```python
from build123d import *

# Parameters (mm, degrees)
BASE_SKETCH_W           = 304.8
BASE_SKETCH_H           = 191.39
BOSS_EXTRUDE1_DEPTH     = 11.81
JOINT_X_W               = 25.4
JOINT_X_H               = 11.81
BOSS_EXTRUDE2_DEPTH     = 11.81
JOINT_Y_W               = 11.81
JOINT_Y_H               = 25.4
CUT_EXTRUDE1_DEPTH      = 384.912686042
LPATTERN1_COUNT         = 4
LPATTERN1_PITCH         = 93.133333333
LPATTERN2_COUNT         = 4
LPATTERN2_PITCH         = 59.266666667
MIRROR1_COPY_1_SKETCH_W = 11.81
MIRROR1_COPY_1_SKETCH_H = 25.4
MIRROR1_COPY_1_DEPTH    = 384.912686042
MIRROR1_COPY_2_SKETCH_W = 11.81
MIRROR1_COPY_2_SKETCH_H = 25.4
MIRROR1_COPY_2_DEPTH    = 384.912686042
MIRROR1_COPY_3_SKETCH_W = 11.81
MIRROR1_COPY_3_SKETCH_H = 25.4
MIRROR1_COPY_3_DEPTH    = 384.912686042


with BuildPart() as part:
    # Base_Sketch → Boss-Extrude1 (new body)
    with BuildSketch(Plane.XY):
        with Locations((-199.719002607, -45.012810132)):
            Rectangle(BASE_SKETCH_W, BASE_SKETCH_H)
    extrude(amount=BOSS_EXTRUDE1_DEPTH)

    # Joint_X → Boss-Extrude2 (add)
    with BuildSketch(Plane.XY.offset(11.81)):
        with Locations((-339.419002607, -146.612810132)):
            Rectangle(JOINT_X_W, JOINT_X_H)
    boss_extrude2 = extrude(amount=-BOSS_EXTRUDE2_DEPTH)

    # Joint_Y → Cut-Extrude1 (cut, through all)
    with BuildSketch(Plane.XY.offset(11.81)):
        with Locations((-346.214002607, -139.817810132)):
            Rectangle(JOINT_Y_W, JOINT_Y_H)
    cut_extrude1 = extrude(amount=-CUT_EXTRUDE1_DEPTH, mode=Mode.SUBTRACT)

    # LPattern1: Boss-Extrude2 ×4
    with Locations(*[(i * LPATTERN1_PITCH, 0, 0) for i in range(1, LPATTERN1_COUNT)]):
        add(boss_extrude2)

    # LPattern2: Cut-Extrude1 ×4
    with Locations(*[(0, i * LPATTERN2_PITCH, 0) for i in range(1, LPATTERN2_COUNT)]):
        add(cut_extrude1, mode=Mode.SUBTRACT)

    # Mirror1: Cut-Extrude1 across plane
    add(cut_extrude1.mirror(Plane.ZY.offset(199.719002607)), mode=Mode.SUBTRACT)

    # Mirror1 copy 1 sketch → Mirror1 copy 1 (cut, through all)
    with BuildSketch(Plane(origin=(-399.438005213, 59.266666667, 11.81), x_dir=(-1, 0, 0), z_dir=(0, 0, 1))):
        with Locations((-346.214002607, 139.817810132)):
            Rectangle(MIRROR1_COPY_1_SKETCH_W, MIRROR1_COPY_1_SKETCH_H)
    extrude(amount=-MIRROR1_COPY_1_DEPTH, mode=Mode.SUBTRACT)

    # Mirror1 copy 2 sketch → Mirror1 copy 2 (cut, through all)
    with BuildSketch(Plane(origin=(-399.438005213, 118.533333333, 11.81), x_dir=(-1, 0, 0), z_dir=(0, 0, 1))):
        with Locations((-346.214002607, 139.817810132)):
            Rectangle(MIRROR1_COPY_2_SKETCH_W, MIRROR1_COPY_2_SKETCH_H)
    extrude(amount=-MIRROR1_COPY_2_DEPTH, mode=Mode.SUBTRACT)

    # Mirror1 copy 3 sketch → Mirror1 copy 3 (cut, through all)
    with BuildSketch(Plane(origin=(-399.438005213, 177.8, 11.81), x_dir=(-1, 0, 0), z_dir=(0, 0, 1))):
        with Locations((-346.214002607, 139.817810132)):
            Rectangle(MIRROR1_COPY_3_SKETCH_W, MIRROR1_COPY_3_SKETCH_H)
    extrude(amount=-MIRROR1_COPY_3_DEPTH, mode=Mode.SUBTRACT)


solid = part.part
```
Geometry: final body of the model. Coordinates: model frame, mm. A direction names the side the tool comes from. Round coordinates to 2 decimals unless told otherwise and drop trailing zeros. Order: outer loops, then holes, each group sorted by start corner. A loop starts at its lowest first (then second) coordinate and runs counter-clockwise, first axis right, second up. Notation, with made-up numbers: (43, -11) - (100, -11) arc R30 cw to (100, 19) - close; hole circle Ø6 at (-33.75, 78.5). An arc over 180 degrees is marked (long way). Write item = value, one per line. Start each with the question number.
Q1. Cut plane B-B on y = -80. Return the cut outline in (x, z), and give its area (3 significant figures).
Q2. Cut plane A-A on x = -189.5. Return the cut outline in (y, z).
Q3. Pin query (flat end, axial travel): pin 1 (3.5 mm diameter, centred on x = -344.5, z = 5.5, fed in from +Y); pin 2 (6 mm diameter, centred on x = -343.5, z = 4, fed in from -Y); pin 3 (3.5 mm diameter, centred on y = -149, z = 8, fed in from +X). Return the tip coordinate at first contact, or that it passes through.
Q4. Pull-direction query (X, two-part tool) for faces 4 (the flat face through (-53, -127.118, 6)), 5 (the flat face through (-293, -140.708, 6)), 6 (the flat face through (-352.119, -51, 6)); classes: +X half, -X half, draft (parallel to the pull), parting line (faces both ways), or undercut.
Q5. Access query for faces 1 (the flat face through (-346, 25.282, 6)), 2 (the flat face through (-107, -140.708, 6)), 3 (the flat face through (-59.129, 38, 6)). Directions: +Z, -Z, +X, -X, +Y, -Y. A direction counts if a zero-diameter tool reaches every point of the face in a straight line with its end or side. Return the directions, or none.
Q6. Ray query, line 1 (X direction, y = -131.5, z = 11); line 2 (Y direction, x = -188, z = 5.25). Return the intervals inside material, ascending. Write a range as from..to.
Outcome:
q1.outline = (-340.31, 0) - (-59.13, 0) - (-59.13, 11.81) - (-340.31, 11.81) - close
q1.area = 3,320 mm^2
q2.outline = (-140.71, 0) - (50.68, 0) - (50.68, 11.81) - (-140.71, 11.81) - close
q3.pin_1 = 25.28
q3.pin_2 = -127.12
q3.pin_3 = -59.13
q4.face_4 = draft
q4.face_5 = undercut
q4.face_6 = -X half
q5.face_1 = +Z, -Z, -X, +Y
q5.face_2 = +Z, -Z, -Y
q5.face_3 = +Z, -Z, +X, +Y
q6.line_1 = -340.31..-59.13
q6.line_2 = -140.71..50.68
